Here's how the part is built. I have some questions about the finished solid (model axes, mm). A direction names the side the tool comes from. Give positions to 0.01 mm unless a question says otherwise; leave off trailing zeros. Write each loop counter-clockwise with the first axis right and the second up, starting at its lowest first coordinate (ties: lowest second). Pieces come first, ordered by that corner, then holes. Notation, with made-up numbers: (37.5, 15.25) - (84.5, 15.25) arc R34 ccw to (84.5, 45.25) - close; hole circle Ø6 at (-21.75, 79). An arc over 180 degrees is marked (long way). Use a Markdown table: item, result.
```python
from build123d import *

# Parameters (mm, degrees)
SKETCH2_W             = 22.718450652
SKETCH2_H             = 2.54
EXTRUDE_THIN1_DEPTH   = 30.48
SKETCH2_W_2           = 2.54
SKETCH2_H_2           = 25.4
EXTRUDE_THIN1_2_DEPTH = 30.48
CHAMFER1_SIZE         = 1.27


with BuildPart() as part:
    # Sketch2 → Extrude-Thin1 (new, symmetric)
    with BuildSketch(Plane(origin=(0, 0, 0), x_dir=(1, 0, 0), z_dir=(0, 1, 0))):
        Rectangle(SKETCH2_W, SKETCH2_H)
    extrude(amount=EXTRUDE_THIN1_DEPTH, both=True)


with BuildPart() as body_2:
    # Sketch2 → Extrude-Thin1 2 (new, symmetric)
    with BuildSketch(Plane(origin=(0, 0, 0), x_dir=(1, 0, 0), z_dir=(0, 1, 0))):
        with Locations((0, 12.7)):
            Rectangle(SKETCH2_W_2, SKETCH2_H_2)
    extrude(amount=EXTRUDE_THIN1_2_DEPTH, both=True)

    # Combine1: union part
    add(part.part)

    # Chamfer1
    chamfer1_edges = [body_2.edges().sort_by_distance(p)[0] for p in [
        (-11.359225326, 0, 1.27),
        (11.359225326, 0, 1.27),
        (1.27, 0, -25.4),
        (-1.27, 0, -25.4),
    ]]
    chamfer(chamfer1_edges, length=CHAMFER1_SIZE - 0.0001)  # a hair under: the kernel refuses the full size


solid = body_2.part
```
Item 1: For faces 4 (the flat face through (1.27, 0, -13)), 5 (the flat face through (-1.27, 0, -13)), 6 (the flat face through (-10.72, -0.43, 0.64)), which set-ups out of +Z, -Z, +X, -X, +Y, -Y let a thin tool reach every point of the face, with its end or its side?
Values:
| item | result |
|---|---|
| face 4 | -Z, +X, +Y, -Y |
| face 5 | -Z, -X, +Y, -Y |
| face 6 | +Z, -X, +Y, -Y |
Item 2: Will these pins go through, and if not, where does the flat tip stop? pin 1 Ø10 at (y, z) = (5, -16.5) entering from +X; pin 2 Ø3 at (y, z) = (10, -5.5) entering from -X; pin 3 Ø5 at (x, y) = (7.5, -4) entering from -Z.
Values:
| item | result |
|---|---|
| pin 1 | stops at x = 1.27 |
| pin 2 | stops at x = -1.27 |
| pin 3 | stops at z = -1.27 |
Item 3: I need wall thicknesses on line 1 along Z through (x, y) = (6.25, -6.5); line 2 along Z through (x, y) = (0.75, 20). Which ranges of each line are inside material? Lowest first, please. Write a range as [from, to].
Values:
| item | result |
|---|---|
| line 1 | z = [-1.27, 1.27] |
| line 2 | z = [-24.65, 1.27] |
Item 4: If we section it at C-C, the plane x = 4.75: Write out the boundary of the cut face in (y, z).
Values:
| item | result |
|---|---|
| outline | (-30.48, -1.27) - (30.48, -1.27) - (30.48, 1.27) - (-30.48, 1.27) - close |
Item 5: Thinking about a two-plate mould opening in X: for faces 1 (the flat face through (10.73, -0.43, 0.63)), 2 (the flat face through (-11.359, 0, -1)), 3 (the flat face through (0, 30.48, -6)), which applies, +X half, -X half, draft (parallel to the pull), parting line (faces both ways), or undercut?
Values:
| item | result |
|---|---|
| face 1 | +X half |
| face 2 | -X half |
| face 3 | draft |
Item 6: If we section it at B-B, the plane z = -10.75: Write out the boundary of the cut face in (x, y).
Values:
| item | result |
|---|---|
| outline | (-1.27, -30.48) - (1.27, -30.48) - (1.27, 30.48) - (-1.27, 30.48) - close |
